Part model, mm, in its own coordinate system. Face numbers are marked on the shaded views. A direction names the side the tool comes from. Give positions to 0.01 mm unless a question says otherwise; leave off trailing zeros. Loops run counter-clockwise (first coordinate to the right, second up) from the corner with the lowest first, then second, coordinate; pieces in that order, holes last. Notation, with made-up numbers: (26, 9.5) -> (42, 9.5) arc R25 cw to (42, 40.5) -> close; hole circle Ø4 at (28, -16). An arc over 180 degrees is marked (long way). Write item = value, one per line.
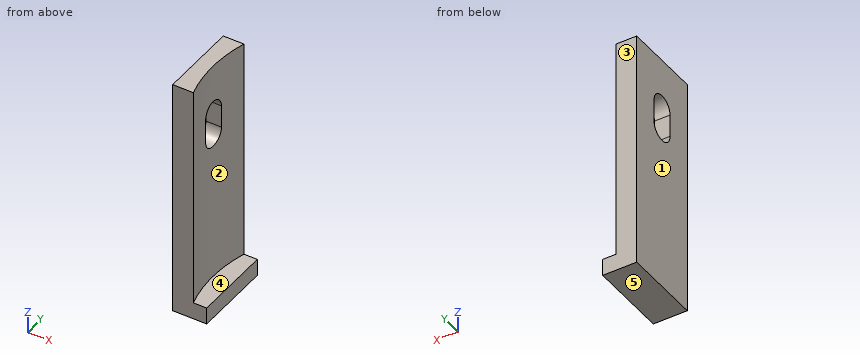
from build123d import *

# Parameters (mm, degrees)
BOX_W             = 6
BOX_H             = 14
BOX_DEPTH         = 42.5
POCKET077_DEPTH   = 28.001
CYLINDER012_R     = 25.35
CYLINDER012_DEPTH = 51.142136


with BuildPart() as part:
    # Box → Box (join)
    with BuildSketch(Plane(origin=(-28, -7, -42.142136), x_dir=(1, 0, 0), z_dir=(0, 0, 1))):
        with Locations((3, 7)):
            Rectangle(BOX_W, BOX_H)
    extrude(amount=BOX_DEPTH)

    # Sketch136 → Pocket077 (cut, through all)
    with BuildSketch(Plane.YZ):
        with BuildLine():
            ThreePointArc((2.2, -8.5), (0, -6.3), (-2.2, -8.5))
            Line((-2.2, -8.5), (-2.2, -12.5))
            ThreePointArc((-2.2, -12.5), (0, -14.7), (2.2, -12.5))
            Line((2.2, -8.5), (2.2, -12.5))
        make_face()
    extrude(amount=-POCKET077_DEPTH, mode=Mode.SUBTRACT)

    # Cylinder012 → Cylinder012 (cut)
    with BuildSketch(Plane.XY.offset(-39.142136)):
        Circle(CYLINDER012_R)
    extrude(amount=CYLINDER012_DEPTH, mode=Mode.SUBTRACT)


with BuildPart() as part_1:
    # Body022028 placement: moved
    add(part.part.moved(Location((-2.5, 0, 848.142136))))


solid = part_1.part
1) Drill centre lines: line 1 along Z through (x, y) = (-25.5, 4.75); line 2 along Z through (x, y) = (-28.25, 1.25); line 3 along Z through (x, y) = (-29, -1). Where is each one in solid material? Low to high. Write a range as [from, to].
Resolved:
line_1 = [806, 809]
line_2 = [806, 833.83], [841.45, 848.5]
line_3 = [806, 833.68], [841.6, 848.5]
2) Slice it at C-C, the plane z = 836.5. List the corners of the cut face in (x, y).
Resolved:
outline = (-30.5, -7) -> (-26.86, -7) arc R25.35 cw to (-27.75, -2.2) -> (-30.5, -2.2) -> close; (-30.5, 2.2) -> (-27.75, 2.2) arc R25.35 cw to (-26.86, 7) -> (-30.5, 7) -> close
3) Slice it at A-A, the plane y = 0. List the corners of the cut face in (x, z), and give its area (3 significant figures).
Resolved:
outline = (-30.5, 806) -> (-24.5, 806) -> (-24.5, 809) -> (-27.85, 809) -> (-27.85, 833.44) -> (-30.5, 833.44) -> close; (-30.5, 841.84) -> (-27.85, 841.84) -> (-27.85, 848.5) -> (-30.5, 848.5) -> close
area = 100 mm²
4) Slice it at B-B, the plane x = -29.25. List the corners of the cut face in (y, z).
Resolved:
outline = (-7, 806) -> (7, 806) -> (7, 848.5) -> (-7, 848.5) -> close; hole (-2.2, 835.64) arc R2.2 ccw to (2.2, 835.64) -> (2.2, 839.64) arc R2.2 ccw to (-2.2, 839.64) -> close
5) Pull direction Y, two halves, no side cores. Call the marked faces 3, 4 and 5: pulls with the +Y half, pulls with the -Y half, needs draft (parallel to the pull), parting line crosses it, or undercut.
Resolved:
face_3 = pulls with the +Y half
face_4 = undercut
face_5 = needs draft
6) Which spindle directions (+Z, -Z, +X, -X, +Y, -Y) get a long thin tool onto all of the face, cutting with end or side? Do the marked faces 1 and 2. Say none if no direction does.
Resolved:
face_1 = +Z, -Z, -X, +Y, -Y
face_2 = +Z, +X
7) Slice it at D-D, the plane z = 831. List the corners of the cut face in (x, y), and give its area (3 significant figures).
Resolved:
outline = (-30.5, -7) -> (-26.86, -7) arc R25.35 cw to (-26.86, 7) -> (-30.5, 7) -> close
area = 41.7 mm²
8) Drop a flat-ended pin along its axis: P1, Ø1.7, axis at x = -25.5, y = 3.5, coming from the +Z side. Give the stop position or say it passes through.
Resolved:
P1 = 809
